Geometry: final body of the model. Coordinates: model frame, mm. Give positions to 0.01 mm unless a question says otherwise; leave off trailing zeros. Write each loop counter-clockwise with the first axis right and the second up, starting at its lowest first coordinate (ties: lowest second). Pieces come first, ordered by that corner, then holes. Notation, with made-up numbers: M 72.5,31 L 122.5,31 A26 cw 122.5,46 Z; hole C -13,56.25 d11. An arc over 180 degrees is marked long. Use one line per item in the form item = value. Start each with the question number.
Item 1: Section query B-B on y = 40. Return loops of the section in (x, z), then the cut area to 3 significant figures.
Item 2: Section query A-A on x = 19. Return loops of the section in (y, z).
Item 3: Material intervals for line 1 along Y through (x, z) = (19, 2.45); line 2 along X through (y, z) = (44.5, 0.65); line 3 along X through (y, z) = (37.5, 2.85), sorted ascending. Write a range as from..to.
Item 4: Section query D-D on y = -40. Return loops of the section in (x, z), then the cut area to 3 significant figures.
Item 5: Section query C-C on z = 2.1. Return loops of the section in (x, y), then the cut area to 3 significant figures.
Item 6: Contact query for a flat-ended pin moving along its axis: P1, Ø6.5, axis at x = 19, y = -40, coming from the -Z side. Output: stop coordinate, or through.
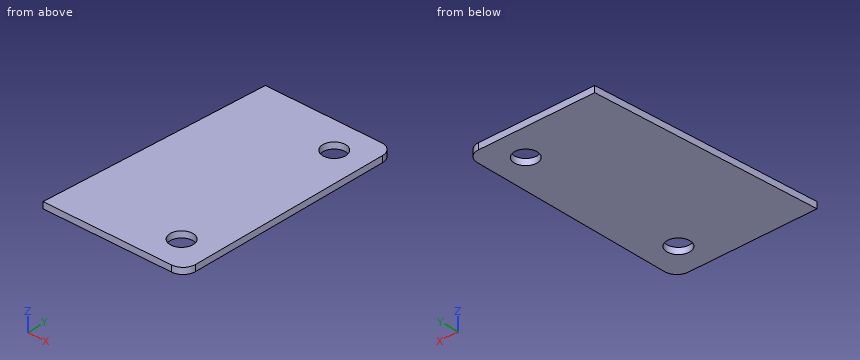
Autodesk Inventor part; units mm, degrees
ref_plane "YZ Plane" through (0, 0, 0) normal (1, 0, 0) x (0, 1, 0)
ref_plane "XZ Plane" through (0, 0, 0) normal (0, 1, 0) x (-1, 0, 0)
ref_plane "XY Plane" through (0, 0, 0) normal (0, 0, 1) x (1, 0, 0)
sketch "Sketch1" plane through (0, 0, 0) normal (0, 0, 1) x (1, 0, 0)
  line L0 (-34, 55) -> (34, 55)
  line L1 (34, 55) -> (34, -55)
  line L2 (34, -55) -> (-34, -55)
  line L3 (-34, -55) -> (-34, 55)
  line L4 (-34, 55) -> (34, -55) construction
  line L5 (34, 55) -> (-34, -55) construction
  line L6 (-34, -19) -> (-34, 19)
  circle A0 centre (19, 40) radius 5.5
  circle A1 centre (19, -40) radius 5.5
  line L7 (0, 0) -> (34, 0) construction
  line L8 (-34, -55) -> (-28, 55)
  dimension "d157" = 68
  dimension "d158" = 110
  dimension "d160" = 80
  dimension "d161" = 11
  dimension "d164" = 15
  dimension "d165" = 6
extrude "Plate3" add sketch "Sketch1" along normal blind 3 contours L0 L1 L2 L8
fillet "Corner Round2" radius 6 2 edges at (34, 55, 1.5) (34, -55, 1.5)
equation "\"BendReliefWidth\" = Thickness"
equation "\"BendReliefDepth\" = 0.5 * Thickness"
equation "\"CornerReliefSize\" = 4 * Thickness"
equation "\"MinimumRemnant\" = 2 * Thickness"
equation "\"GapSize\" = Thickness"
properties part number "MSC 815 wall inner joint" material "AISI304"
Answer sheet:
q1.outline = M -28.82,0 L 13.5,0 L 13.5,3 L -28.82,3 Z; M 24.5,0 L 34,0 L 34,3 L 24.5,3 Z
q1.area = 155 mm2
q2.outline = M -55,0 L -45.5,0 L -45.5,3 L -55,3 Z; M -34.5,0 L 34.5,0 L 34.5,3 L -34.5,3 Z; M 45.5,0 L 55,0 L 55,3 L 45.5,3 Z
q3.line_1 = -55..-45.5, -34.5..34.5, 45.5..55
q3.line_2 = -28.57..15.84, 22.16..34
q3.line_3 = -28.95..14.1, 23.9..34
q4.outline = M -33.18,0 L 13.5,0 L 13.5,3 L -33.18,3 Z; M 24.5,0 L 34,0 L 34,3 L 24.5,3 Z
q4.area = 169 mm2
q5.outline = M -34,-55 L 28,-55 A6 ccw 34,-49 L 34,49 A6 ccw 28,55 L -28,55 Z; hole C 19,-40 d11; hole C 19,40 d11
q5.area = 6,940 mm2
q6.P1 = through
